Autodesk Inventor part; units mm, degrees
ref_plane "YZ Plane" through (0, 0, 0) normal (1, 0, 0) x (0, 1, 0)
ref_plane "XZ Plane" through (0, 0, 0) normal (0, 1, 0) x (-1, 0, 0)
ref_plane "XY Plane" through (0, 0, 0) normal (0, 0, 1) x (1, 0, 0)
sketch "Sketch1" plane through (0, 0, 0) normal (0, 1, 0) x (-1, 0, 0)
  line L0 (0, 0) -> (80, 0)
  line L1 (80, 0) -> (80, -150)
  line L2 (80, -150) -> (0, -150)
  line L3 (0, -150) -> (0, 0)
  dimension "d0" = 80
  dimension "d1" = 150
extrude "Extrusion1" add sketch "Sketch1" along normal blind 140
sketch "Sketch2" plane through (0, 0, 0) normal (1, 0, 0) x (0, 0, -1)
  line L0 (150, 140) -> (0, 140)
  line L1 (61.0962, 140) -> (61.0962, 100)
  line L2 (61.0962, 100) -> (15.8986, 100)
  line L3 (15.8986, 80) -> (79.9832, 29)
  line L4 (79.9832, 29) -> (79.9832, 14)
  line L5 (79.9832, 14) -> (142.2187, 14)
  line L6 (142.2187, 14) -> (142.2187, 44)
  line L7 (142.2187, 44) -> (150, 44)
  line L8 (150, 0) -> (150, 140)
  line L9 (150, 44) -> (150, 140)
  line L10 (150, 140) -> (61.0962, 140)
  line L11 (15.8986, 100) -> (15.8986, 80)
  line L12 (0, 0) -> (150, 0)
  point P0 (146.1093, 44)
  point P1 (111.101, 14)
  dimension "d7" = 15
  dimension "d8" = 30
  dimension "d9" = 14
  dimension "d11" = 40
  dimension "d12" = 20
extrude "Extrusion2" cut sketch "Sketch2" against normal blind 140
sketch "Sketch3" plane through (0, 14, -79.9832) normal (0, 1, 0) x (1, 0, 0)
  line L0 (0, -79.9832) -> (0, 70.0168)
  line L1 (0, 0) -> (-80, 0)
  line L2 (0, 62.5105) -> (-4, 62.5105)
  line L3 (-4, 62.5105) -> (-4, 0)
  line L4 (-4, 0) -> (0, 0)
  line L5 (0, 0) -> (0, 62.5105)
  dimension "d13" = 4
extrude "Extrusion3" add sketch "Sketch3" along normal blind 15
sketch "Sketch4" plane through (0, 140, 0) normal (0, 1, 0) x (1, 0, 0)
  circle A0 centre (-40, 43.0962) radius 15.5
  line L0 (0, 61.0962) -> (-80, 61.0962)
  line L1 (0, 0) -> (0, 61.0962)
  dimension "d18" = 31
  dimension "d19" = 18
  dimension "d20" = 40
extrude "Extrusion4" cut sketch "Sketch4" against normal blind 50
sketch "Sketch5" plane through (0, 140, 0) normal (0, 1, 0) x (1, 0, 0)
  line L0 (-18, 24) -> (-62, 24)
  line L1 (-62, 24) -> (-62, 60)
  line L2 (-62, 60) -> (-18, 60)
  line L3 (-18, 60) -> (-18, 24)
  line L4 (-80, 61.0962) -> (-80, 0)
  line L5 (0, 0) -> (0, 61.0962)
  line L6 (-80, 0) -> (0, 0)
  line L7 (0, 61.0962) -> (-80, 61.0962)
  dimension "d21" = 36
  dimension "d22" = 18
  dimension "d23" = 18
  dimension "d26" = 24
extrude "Extrusion5" cut sketch "Sketch5" against normal blind 5 contours L0 L1 L2 L3
sketch "Sketch6" plane through (-80, 80, -15.8986) normal (0, 0.7824608, -0.6226999) x (1, 0, 0)
  line L0 (76, 81.9014) -> (0, 81.9014)
  line L1 (8.3307, 81.9014) -> (38, 27.8393)
  line L2 (38, 27.8393) -> (42.4953, 27.8393)
  line L3 (42.4953, 27.8393) -> (12.826, 81.9014)
  line L4 (12.826, 81.9014) -> (8.3307, 81.9014)
  point P0 (80, 37.376)
  point P1 (12.826, 81.9014)
extrude "Extrusion6" add sketch "Sketch6" along normal blind 30
sketch "Sketch7" plane through (-71.6693, 29, -79.9832) normal (-0.8766596, 0.2995878, 0.3764506) x (0.4811111, 0.5458959, 0.6859518)
  line L0 (-0.005, -0.0058) -> (32.9106, 38.0398)
  line L1 (32.9106, 38.0398) -> (9.9736, 41.528)
  line L2 (2.1627, 30) -> (0, 30)
  line L3 (9.9736, 41.528) -> (0, 30)
  line L4 (0, 30) -> (0, 0)
  point P0 (73.5146, -72.4969)
extrude "Extrusion7" cut sketch "Sketch7" against normal blind 15
properties part number "Right"
Model file for the job. Use its own axes, mm. A direction names the side the tool comes from. Round coordinates to 2 decimals unless told otherwise and drop trailing zeros. Write each loop counter-clockwise with the first axis right and the second up, starting at its lowest first coordinate (ties: lowest second). Pieces come first, ordered by that corner, then holes. Notation, with made-up numbers: (-29, 44.5) -> (5, 44.5) arc R16 ccw to (5, 66.5) -> close; hole circle Ø6 at (5, 41). An arc over 180 degrees is marked (long way). Answer as CSV lines item,"result".
1. Tool access for faces 1 (the face through (-50, 135, -30)), 2 (the face through (-4, 21, -112)), 3 (the face through (-48.835, 61.381, -63.046)), 4 (the face through (-2, 29, -112)): list every direction of +Z, -Z, +X, -X, +Y, -Y with a clear straight run to the whole face (end or side of a thin tool).
Resolved:
face 1,"+Y"
face 2,"-X, +Y"
face 3,"+X"
face 4,"+X, -X, +Y"
2. Slice it at C-C, the plane x = -40. List the corners of the cut face in (y, z).
Resolved:
outline,"(0, -150) -> (44, -150) -> (44, -142.22) -> (14, -142.22) -> (14, -79.98) -> (29, -79.98) -> (59.83, -41.24) -> (83.31, -59.92) -> (86.14, -56.36) -> (62.66, -37.68) -> (80, -15.9) -> (100, -15.9) -> (100, -27.6) -> (135, -27.6) -> (135, -24) -> (140, -24) -> (140, 0) -> (0, 0) -> close; (100, -61.1) -> (140, -61.1) -> (140, -60) -> (135, -60) -> (135, -58.6) -> (100, -58.6) -> close"
3. Slice it at D-D, the plane x = -65. List the corners of the cut face in (y, z).
Resolved:
outline,"(0, -150) -> (44, -150) -> (44, -142.22) -> (14, -142.22) -> (14, -79.98) -> (29, -79.98) -> (31.47, -76.88) -> (37.51, -81.69) -> (49.1, -80.45) -> (36.57, -70.47) -> (80, -15.9) -> (100, -15.9) -> (100, -61.1) -> (140, -61.1) -> (140, 0) -> (0, 0) -> close"
4. Pin check, flat tips, straight feed: pin 1 Ø18 at (x, z) = (-41, -37) entering from +Y; pin 2 Ø4.5 at (x, z) = (-2, -102) entering from +Y; pin 3 Ø2 at (x, z) = (-30.5, -106) entering from +Y. Stop position of each tip, or through.
Resolved:
pin 1,"y = 73.12"
pin 2,"y = 29"
pin 3,"y = 14"
5. Drill centre lines: line 1 (Z direction, x = -44, y = 15); line 2 (Z direction, x = -40, y = 115); line 3 (Y direction, x = -16, z = -86.5). Where is each one in solid material? Low to high.
Resolved:
line 1,"-150 to -142.22, -79.98 to 0"
line 2,"-61.1 to -58.6, -27.6 to 0"
line 3,"0 to 14"
6. Slice it at A-A, the plane y = 59. List the corners of the cut face in (x, z), plus the area to 3 significant figures.
Resolved:
outline,"(-80, -42.29) -> (-45.23, -42.29) -> (-61.72, -80.68) -> (-57.87, -82.19) -> (-40.73, -42.29) -> (0, -42.29) -> (0, 0) -> (-80, 0) -> close"
area,"3,560 mm²"
7. Slice it at B-B, the plane z = -129. List the corners of the cut face in (x, y).
Resolved:
outline,"(-80, 0) -> (0, 0) -> (0, 29) -> (-4, 29) -> (-4, 14) -> (-80, 14) -> close"
8. Mould opens along Z. For faces 5 (the face through (-18, 138, -42)), 6 (the face through (-41, 22, -150)), 7 (the face through (-39, 0, -74)), 8 (the face through (-39, 69, 0)) say: +Z half, -Z half, draft (parallel to the pull), parting line (faces both ways), or undercut.
Resolved:
face 5,"undercut"
face 6,"-Z half"
face 7,"draft"
face 8,"+Z half"
